Build history of the part. All positions in model axes, mm. Give positions to 0.01 mm unless a question says otherwise; leave off trailing zeros. Write each loop counter-clockwise with the first axis right and the second up, starting at its lowest first coordinate (ties: lowest second). Pieces come first, ordered by that corner, then holes.
from build123d import *

# Parameters (mm, degrees)
ESQUISSE2_R                  = 78.359
ESQUISSE2_R_2                = 76.2
BOSS_EXTRU_1_DEPTH           = 787.4
ESQUISSE3_W                  = 6.35
ESQUISSE3_H                  = 203.2
ENL_V_MAT_EXTRU_1_DEPTH      = 153.416
R_P_TITION_CIRCULAIRE1_COUNT = 3


with BuildPart() as part:
    # Esquisse2 → Boss.-Extru.1 (new body)
    with BuildSketch(Plane.XY):
        Circle(ESQUISSE2_R)
        Circle(ESQUISSE2_R_2, mode=Mode.SUBTRACT)
    extrude(amount=BOSS_EXTRU_1_DEPTH)

    # Esquisse3 → Enlèv. mat.-Extru.1 (cut)
    with BuildSketch(Plane(origin=(0, 0, 0), x_dir=(1, 0, 0), z_dir=(0, 1, 0))):
        with Locations((0, -673.1)):
            Rectangle(ESQUISSE3_W, ESQUISSE3_H)
    enl_v_mat_extru_1 = extrude(amount=ENL_V_MAT_EXTRU_1_DEPTH, mode=Mode.SUBTRACT)

    # Répétition circulaire1: Enlèv. mat.-Extru.1 ×3 about axis
    r_p_tition_circulaire1_axis = Axis((0, 0, 0), (0, 0, 1))
    for i in range(1, R_P_TITION_CIRCULAIRE1_COUNT):
        add(enl_v_mat_extru_1.rotate(r_p_tition_circulaire1_axis, i * 360 / R_P_TITION_CIRCULAIRE1_COUNT), mode=Mode.SUBTRACT)


solid = part.part
1. Mould opens along X. For faces 1 (the face through (74.74, 23.54, 388.19)), 2 (the face through (17, -75, 787.4)), 3 (the face through (-60.47, -46.367, 388.188)) say: pulls with the +X half, pulls with the -X half, needs draft (parallel to the pull), parting line crosses it, or undercut.
2. Saw through at A-A on y = 0. Give the cut face in (x, z), plus the area to 3 significant figures.
3. Drill centre lines: line 1 along Y through (x, z) = (0, 179); line 2 along Y through (x, z) = (0, 602); line 3 along Y through (x, z) = (48.5, 114). Where is each one in solid material? Low to high.
4. Saw through at B-B on x = 45. Give the cut face in (y, z).
5. Drop flat-ended pins along their axis: pin 1 (3 mm diameter, centred on y = -13, z = 572.5, fed in from -X); pin 2 (1 mm diameter, centred on y = -31.5, z = 265.5, fed in from +X); pin 3 (6 mm diameter, centred on x = 31, z = 486, fed in from -Y). Give the stop position or say it passes through.
6. Saw through at C-C on z = 337. Give the cut face in (x, y).
Outcome:
1. face 1: parting line crosses it
1. face 2: needs draft
1. face 3: undercut
2. outline: (-78.36, 0) - (-76.2, 0) - (-76.2, 787.4) - (-78.36, 787.4) - close; (76.2, 0) - (78.36, 0) - (78.36, 787.4) - (76.2, 787.4) - close
2. area: 3,400 mm2
3. line 1: y = -78.36 to -76.2, 76.2 to 78.36
3. line 2: y = -78.36 to -76.2
3. line 3: y = -61.55 to -58.77, 58.77 to 61.55
4. outline: (-64.15, 0) - (-61.49, 0) - (-61.49, 787.4) - (-64.15, 787.4) - close; (61.49, 0) - (64.15, 0) - (64.15, 787.4) - (61.49, 787.4) - close
5. pin 1: stops at x = -77.51
5. pin 2: stops at x = 71.97
5. pin 3: stops at y = -73.19
6. outline: circle Ø156.72 at (0, 0); hole circle Ø152.4 at (0, 0)
